```python
from build123d import *

# Parameters (mm, degrees)
SKETCH1_R                 = 1.651
BOSS_EXTRUDE2_DEPTH       = 3.048
SKETCH2_R                 = 1.143
CUT_EXTRUDE1_DEPTH        = 4.048
SKETCH3_R                 = 12.1285
CUT_EXTRUDE2_DEPTH        = 4.048
SKETCH4_W                 = 28.562713242
SKETCH4_H                 = 11.677503754
BOSS_EXTRUDE3_DEPTH       = 3.048
SKETCH5_W                 = 230.699333954
SKETCH5_H                 = 107.587024537
CUT_EXTRUDE3_DEPTH        = 4.048
SKETCH6_R                 = 12.1285
CUT_EXTRUDE4_DEPTH        = 4.048
SKETCH9_W                 = 11.43
SKETCH9_H                 = 10.16
CUT_EXTRUDE7_DEPTH        = 4.048
SKETCH65_R                = 1.651
CUT_EXTRUDE63_DEPTH       = 97.79
SKETCH119_R               = 3.175
CUT_EXTRUDE117_DEPTH      = 103.378
CUT_EXTRUDE117_DEPTH_BACK = 48.768
CUT_EXTRUDE10_DEPTH       = 14.224
FILLET1_R                 = 2.54


with BuildPart() as part:
    # Sketch1 → Boss-Extrude2 (new body)
    with BuildSketch(Plane.XY):
        with BuildLine():
            Line((-65.2537815, 36.83), (-54.8397815, 36.83))
            Line((-54.8397815, 36.83), (-54.8397815, -36.83))
            Line((-54.8397815, -36.83), (-65.2537815, -36.83))
            ThreePointArc((-65.2537815, -36.83), (0, -74.93), (65.2537815, -36.83))
            Line((65.2537815, -36.83), (54.8397815, -36.83))
            Line((54.8397815, -36.83), (54.8397815, 36.83))
            Line((54.8397815, 36.83), (65.2537815, 36.83))
            ThreePointArc((65.2537815, 36.83), (0, 74.93), (-65.2537815, 36.83))
        make_face()
        with Locations((-45.466, 11.049)):
            Circle(SKETCH1_R, mode=Mode.SUBTRACT)
        with Locations((-20.067270032, 10.795)):
            Circle(SKETCH1_R, mode=Mode.SUBTRACT)
        with Locations((-20.067270032, -10.795)):
            Circle(SKETCH1_R, mode=Mode.SUBTRACT)
        with Locations((-45.466, -11.049)):
            Circle(SKETCH1_R, mode=Mode.SUBTRACT)
        with Locations((45.466, -11.049)):
            Circle(SKETCH1_R, mode=Mode.SUBTRACT)
        with Locations((20.067270032, -10.795)):
            Circle(SKETCH1_R, mode=Mode.SUBTRACT)
        with Locations((20.067270032, 10.795)):
            Circle(SKETCH1_R, mode=Mode.SUBTRACT)
        with Locations((45.466, 11.049)):
            Circle(SKETCH1_R, mode=Mode.SUBTRACT)
    extrude(amount=BOSS_EXTRUDE2_DEPTH)

    # Sketch2 → Cut-Extrude1 (cut, through all)
    with BuildSketch(Plane.XY.offset(3.048)):
        with Locations((-6.731, 62.23)):
            Circle(SKETCH2_R)
        with Locations((6.731, 62.23)):
            Circle(SKETCH2_R)
    extrude(amount=-CUT_EXTRUDE1_DEPTH, mode=Mode.SUBTRACT)

    # Sketch3 → Cut-Extrude2 (cut, through all)
    with BuildSketch(Plane(origin=(0, 0, 0), x_dir=(-1, 0, 0), z_dir=(0, 0, -1))):
        with Locations((-42.926, -42.926)):
            Circle(SKETCH3_R)
        with Locations((-14.224, 34.29)):
            Circle(SKETCH3_R)
        with Locations((14.224, -34.29)):
            Circle(SKETCH3_R)
        with Locations((14.224, 34.29)):
            Circle(SKETCH3_R)
        with Locations((-42.926, 42.926)):
            Circle(SKETCH3_R)
        with Locations((42.926, 42.926)):
            Circle(SKETCH3_R)
        with Locations((-14.224, -34.29)):
            Circle(SKETCH3_R)
        with Locations((42.926, -42.926)):
            Circle(SKETCH3_R)
    extrude(amount=-CUT_EXTRUDE2_DEPTH, mode=Mode.SUBTRACT)

    # Sketch4 → Boss-Extrude3 (add)
    with BuildSketch(Plane(origin=(0, 0, 0), x_dir=(-1, 0, 0), z_dir=(0, 0, -1))):
        with Locations((-1.488809975, 62.152540216)):
            Rectangle(SKETCH4_W, SKETCH4_H)
    extrude(amount=-BOSS_EXTRUDE3_DEPTH)

    # Sketch5 → Cut-Extrude3 (cut, through all)
    with BuildSketch(Plane(origin=(0, 0, 0), x_dir=(-1, 0, 0), z_dir=(0, 0, -1))):
        with Locations((1.971047261, -36.648512269)):
            Rectangle(SKETCH5_W, SKETCH5_H)
    extrude(amount=-CUT_EXTRUDE3_DEPTH, mode=Mode.SUBTRACT)

    # Sketch6 → Cut-Extrude4 (cut, through all)
    with BuildSketch(Plane(origin=(0, 0, 0), x_dir=(-1, 0, 0), z_dir=(0, 0, -1))):
        with Locations((-15.777608989, 58.882838371)):
            Circle(SKETCH6_R)
        with Locations((15.777608989, 58.882838371)):
            Circle(SKETCH6_R)
    extrude(amount=-CUT_EXTRUDE4_DEPTH, mode=Mode.SUBTRACT)

    # Sketch9 → Cut-Extrude7 (cut, through all)
    with BuildSketch(Plane(origin=(0, 0, 0), x_dir=(-1, 0, 0), z_dir=(0, 0, -1))):
        with Locations((33.8847815, 22.225)):
            Rectangle(SKETCH9_W, SKETCH9_H)
        with Locations((-33.8847815, 22.225)):
            Rectangle(SKETCH9_W, SKETCH9_H)
    extrude(amount=-CUT_EXTRUDE7_DEPTH, mode=Mode.SUBTRACT)

    # Sketch65 → Cut-Extrude63 (cut)
    with BuildSketch(Plane(origin=(30.092005081, 4.08352975, -16.1925), x_dir=(-1, 0, 0), z_dir=(0, 0, -1))):
        with Locations((4.154396091, 41.38247025)):
            Circle(SKETCH65_R)
        with Locations((56.02961407, 41.38247025)):
            Circle(SKETCH65_R)
    extrude(amount=-CUT_EXTRUDE63_DEPTH, mode=Mode.SUBTRACT)

    # Sketch119 → Cut-Extrude117 (cut, two sides)
    with BuildSketch(Plane(origin=(30.092005081, 4.08352975, 19.939), x_dir=(-1, 0, 0), z_dir=(0, 0, -1))) as cut_extrude117_sk:
        with Locations((-16.897994919, 21.31647025)):
            Circle(SKETCH119_R)
        with Locations((77.082005081, 21.31647025)):
            Circle(SKETCH119_R)
        with Locations((30.092005081, 21.31647025)):
            Circle(SKETCH119_R)
    extrude(amount=CUT_EXTRUDE117_DEPTH, mode=Mode.SUBTRACT)
    extrude(cut_extrude117_sk.sketch, amount=-CUT_EXTRUDE117_DEPTH_BACK, mode=Mode.SUBTRACT)

    # Sketch12 → Cut-Extrude10 (cut)
    with BuildSketch(Plane(origin=(0, 0, 0), x_dir=(-1, 0, 0), z_dir=(0, 0, -1))):
        with BuildLine():
            Line((12.7, 20.24), (8.888991966, 20.24))
            ThreePointArc((8.888991966, 20.24), (5.715, 23.495), (2.541008034, 20.24))
            Line((2.541008034, 20.24), (-2.541008034, 20.24))
            ThreePointArc((-2.541008034, 20.24), (-5.715, 23.495), (-8.888991966, 20.24))
            Line((-8.888991966, 20.24), (-12.7, 20.24))
            ThreePointArc((-12.7, 20.24), (-16.235533906, 11.704466094), (-7.7, 15.24))
            Line((-7.7, 15.24), (7.7, 15.24))
            ThreePointArc((7.7, 15.24), (16.235533906, 11.704466094), (12.7, 20.24))
        make_face()
    extrude(amount=-CUT_EXTRUDE10_DEPTH, mode=Mode.SUBTRACT)

    # Fillet1
    fillet1_edges = [part.edges().sort_by_distance(p)[0] for p in [
        (-39.5997815, 17.145, 1.524),
        (-28.1697815, 17.145, 1.524),
        (28.1697815, 17.145, 1.524),
        (39.5997815, 17.145, 1.524),
        (-17.322875188, 17.145, 1.524),
        (17.322875188, 17.145, 1.524),
        (8.888991966, 20.24, 1.524),
        (2.541008034, 20.24, 1.524),
        (-2.541008034, 20.24, 1.524),
        (-8.888991966, 20.24, 1.524),
    ]]
    fillet(fillet1_edges, radius=FILLET1_R)


solid = part.part
```
Could you check a few things on this model? Use its own coordinates, in mm. A direction names the side the tool comes from. Coordinates: 2 decimals unless noted, no trailing zeros. Order: outer loops, then holes, each group sorted by start corner. A loop starts at its lowest first (then second) coordinate and runs counter-clockwise, first axis right, second up. Notation, with made-up numbers: M 75.5,2.5 L 130.5,2.5 A15 cw 130.5,28.5 Z; hole C -13.75,6.25 d5. An arc over 180 degrees is marked long. Use a Markdown table: item, result. Add a question column.
Q1. I want a section at C-C on y = 40. List the corners of the cut face in (x, z) for me.
Q2. Which directions (+Z, -Z, +X, -X, +Y, -Y) give clear straight access to the entire face, cutting with the end or side of a thin tool? Please do faces 5 (the cylindrical face through (-14.994, 19.682, 1.503)), 6 (the cylindrical face through (-48.697, 28.077, 1.545)).
Q3. I want a section at B-B on x = -15. List the corners of the cut face in (y, z) for me, then the cut area to 3 significant figures.
Q4. I want a section at D-D on y = 25.4. Give the number of separate pieces and of enclosed holes in the cut face, then the cut area to 3 significant figures.
Q5. I'm going to push flat-ended pins straight in: pin 1 (1 mm diameter, centred on x = -2.5, z = 1, fed in from +Y); pin 2 (0.6 mm diameter, centred on x = 0, z = 2, fed in from -Y); pin 3 (1.5 mm diameter, centred on x = 61.5, z = 2, fed in from -Y). Where does each tip first touch, or does it pass through?
Q6. I want a section at A-A on y = 65.5. List the corners of the cut face in (x, z) for me.
Q7. If I drill on L1, parallel to X at y = 50.5, z = 0.8; L2, parallel to Y at x = -9, z = 0.3; L3, parallel to Y at x = -46.99, z = 2.25 (3 decimals), over which ranges is the centre line in solid material (lowest first)?
Q8. We'd pull the mould along Y, two halves only. Please class faces 1 (the cylindrical face through (3.02, 29.645, 1.503)), 2 (the cylindrical face through (9.535, 20.621, 1.545)), 3 (the cylindrical face through (-14.2, 70.91, 1.5)), 4 (the flat face through (54.84, 27, 2)): pulls with the +Y half, pulls with the -Y half, needs draft (parallel to the pull), parting line crosses it, or undercut.
Checked values:
| question | item | result |
|---|---|---|
| 1 | outline | M -63.36,0 L -54.7,0 L -54.7,3.05 L -63.36,3.05 Z; M -31.16,0 L -24.92,0 L -24.92,3.05 L -31.16,3.05 Z; M -3.52,0 L 3.52,0 L 3.52,3.05 L -3.52,3.05 Z; M 24.92,0 L 31.16,0 L 31.16,3.05 L 24.92,3.05 Z; M 54.7,0 L 63.36,0 L 63.36,3.05 L 54.7,3.05 Z |
| 2 | face 5 | +Z, -Z, -Y |
| 2 | face 6 | +Z, -Z |
| 3 | outline | M 19.68,0 L 22.19,0 L 22.19,3.05 L 19.68,3.05 Z; M 46.39,0 L 46.78,0 L 46.78,3.05 L 46.39,3.05 Z; M 70.99,0 L 73.41,0 L 73.41,3.05 L 70.99,3.05 Z |
| 3 | area | 16.2 mm² |
| 4 | separate pieces | 8 |
| 4 | enclosed holes | 0 |
| 4 | area | 106 mm² |
| 5 | pin 1 | y = 74.9 |
| 5 | pin 2 | y = 20.24 |
| 5 | pin 3 | y = 36.83 |
| 6 | outline | M -36.39,0 L -25.94,0 L -25.94,3.05 L -36.39,3.05 Z; M -5.61,0 L 5.61,0 L 5.61,3.05 L -5.61,3.05 Z; M 25.94,0 L 36.39,0 L 36.39,3.05 L 25.94,3.05 Z |
| 7 | L1 | -55.36 to -52.4, -33.45 to -24.54, -7.01 to 7.01, 24.54 to 33.45, 52.4 to 55.36 |
| 7 | L2 | 21.06 to 23.34, 45.24 to 48.82, 68.94 to 74.39 |
| 7 | L3 | 17.145 to 22.225, 28.575 to 31.499, 54.353 to 58.365 |
| 8 | face 1 | undercut |
| 8 | face 2 | pulls with the -Y half |
| 8 | face 3 | undercut |
| 8 | face 4 | needs draft |
